Model file for the job. Use its own axes, mm. Face numbers are marked on the shaded views. A direction names the side the tool comes from. Give positions to 0.01 mm unless a question says otherwise; leave off trailing zeros. Loops run counter-clockwise (first coordinate to the right, second up) from the corner with the lowest first, then second, coordinate; pieces in that order, holes last. Notation, with made-up numbers: M 31,-39 L 88,-39 A26 cw 88,-11 Z; hole C 87.5,-12.75 d6. An arc over 180 degrees is marked long. Answer in a Markdown table with one row per item.
Autodesk Inventor part; units mm, degrees
ref_plane "YZ Plane" through (0, 0, 0) normal (1, 0, 0) x (0, 1, 0)
ref_plane "XZ Plane" through (0, 0, 0) normal (0, 1, 0) x (-1, 0, 0)
ref_plane "XY Plane" through (0, 0, 0) normal (0, 0, 1) x (1, 0, 0)
sketch "Sketch1" plane through (0, 0, 0) normal (0, 0, 1) x (1, 0, 0)
  line L0 (-119.142, 1.6299) -> (13.858, 1.6299)
  line L1 (14.858, 0.6299) -> (14.858, -42.3701)
  line L2 (13.858, -43.3701) -> (-119.142, -43.3701)
  line L3 (-120.142, -42.3701) -> (-120.142, 0.6299)
  arc A0 (-119.142, 1.6299) -> (-120.142, 0.6299) centre (-119.142, 0.6299) ccw
  arc A1 (-120.142, -42.3701) -> (-119.142, -43.3701) centre (-119.142, -42.3701) ccw
  arc A2 (13.858, -43.3701) -> (14.858, -42.3701) centre (13.858, -42.3701) ccw
  arc A3 (14.858, 0.6299) -> (13.858, 1.6299) centre (13.858, 0.6299) ccw
  circle A4 centre (8.858, -4.3701) radius 1.5
  circle A5 centre (-87.642, -37.3701) radius 1.5
  circle A6 centre (-75.642, -37.3701) radius 1.5
  circle A7 centre (8.858, -37.3701) radius 1.5
  circle A8 centre (-87.642, -4.3701) radius 1.5
  circle A9 centre (-75.642, -4.3701) radius 1.5
  point P0 (0, 0)
  point P1 (-120.142, 1.6299)
  point P2 (14.858, 1.6299)
  dimension "d0" = 135
  dimension "d2" = 1
  dimension "d3" = 1
  dimension "d7" = 3
  dimension "d8" = 6
  dimension "d9" = 6
  dimension "d10" = 3
  dimension "d11" = 3
  dimension "d14" = 3
  dimension "d15" = 6
  dimension "d16" = 6
  dimension "d17" = 6
  dimension "d18" = 6
  dimension "d19" = 12
  dimension "d20" = 32.5
  dimension "d21" = 3
  dimension "d22" = 3
  dimension "d23" = 6
  dimension "d24" = 6
  dimension "d25" = 32.5
  dimension "d26" = 12
extrude "Extrusion1" add sketch "Sketch1" along normal blind 1
sketch "Sketch2" plane through (14.858, -42.3701, 0) normal (1, 0, 0) x (0, 0, -1)
  line L0 (0, 44) -> (-1, 44)
  line L1 (-25, -1) -> (0, -1)
  line L2 (0, -1) -> (0, 44)
  line L3 (0, 44) -> (-25, 44)
  line L4 (-25, 44) -> (-25, -1)
  line L5 (0, 0) -> (0, -1)
  line L6 (0, -1) -> (-10, -1)
  line L7 (-10, -1) -> (-10, 44)
  line L8 (-10, 44) -> (0, 44)
  line L9 (0, 44) -> (0, -1)
  line L10 (0, -1) -> (-1, -1)
  line L11 (-1, -1) -> (-1, 44)
  line L12 (-1, 44) -> (0, 44)
  line L13 (0, 44) -> (0, -1)
  line L14 (-1, 0) -> (-1, 43)
  line L15 (-10, 9) -> (-1, 9)
  line L16 (-1, 9) -> (-1, 29)
  line L17 (-1, 29) -> (-10, 29)
  line L18 (-10, 29) -> (-10, 9)
  line L19 (-25, 5) -> (-10, 5)
  line L20 (-10, 5) -> (-10, 30)
  line L21 (-10, 30) -> (-25, 30)
  line L22 (-25, 30) -> (-25, 5)
  point P0 (0, 42.3701)
  point P1 (-1, 9)
  dimension "d29" = 25
  dimension "d30" = 10
  dimension "d31" = 10
  dimension "d32" = 20
  dimension "d33" = 6
  dimension "d34" = 25
extrude "Extrusion2" add sketch "Sketch2" against normal blind 1 contours L11 L17 L7 L3 | L7 L21 L4 L3 | L1 L7 L15 L11 | L1 L4 L19 L7
sketch "Sketch3" plane through (-119.142, -43.3701, 0) normal (0, -1, 0) x (1, 0, 0)
  line L0 (0, 0) -> (-1, 0)
  line L1 (134, 25) -> (134, 10)
  line L2 (-1, 0) -> (134, 0)
  line L3 (134, 0) -> (134, 25)
  line L4 (134, 25) -> (-1, 25)
  line L5 (-1, 25) -> (-1, 0)
  point P0 (119.142, 0)
extrude "Extrusion3" add sketch "Sketch3" against normal blind 1
sketch "Sketch4" plane through (-119.142, 1.6299, 0) normal (0, 1, 0) x (1, 0, 0)
  line L0 (134, -25) -> (134, -10)
  line L1 (-1, 0) -> (-1, -1)
  line L2 (134, -25) -> (-1, -25)
  line L3 (-1, -25) -> (-1, 0)
  line L4 (-1, 0) -> (134, 0)
  line L5 (134, 0) -> (134, -25)
  point P0 (119.142, 0)
sketch "Sketch5" plane through (-120.142, -43.3701, 0) normal (-1, 0, 0) x (0, 0, 1)
  line L0 (25, 45) -> (1, 45)
  line L1 (0, 44) -> (0, 0)
  line L2 (25, 45) -> (0, 45)
  line L3 (0, 45) -> (0, 0)
  line L4 (0, 0) -> (25, 0)
  line L5 (25, 0) -> (25, 45)
  circle A0 centre (8, 33) radius 2
  circle A1 centre (8, 8) radius 2
  point P0 (0, 43.3701)
  point P1 (1, 45)
  dimension "d39" = 25
  dimension "d40" = 12
  dimension "d42" = 8
  dimension "d47" = 4
  dimension "d48" = 4
  dimension "d49" = 8
extrude "Extrusion4" add sketch "Sketch5" against normal blind 2
extrude "Extrusion5" add sketch "Sketch4" against normal blind 1
properties part number "arduino mould"
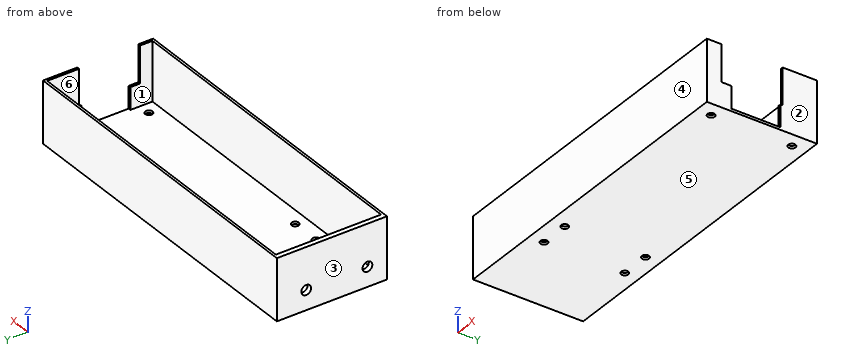
Q1. Probe probe 1 along Y at (x, z) = (-118.7, 8); probe 2 along X at (y, z) = (-5, 21); probe 3 along Y at (x, z) = (-72.5, 1.75). List the from-to ranges inside material, lowest first.
Reported:
| item | result |
|---|---|
| probe 1 | -43.37 to -37.37, -33.37 to -12.37, -8.37 to 1.63 |
| probe 2 | -120.14 to -118.14, 13.86 to 14.86 |
| probe 3 | -43.37 to -42.37, 0.63 to 1.63 |
Q2. Saw through at A-A (z = 8). Give the cut face in (x, y).
Reported:
| item | result |
|---|---|
| outline | M -120.14,-43.37 L 14.86,-43.37 L 14.86,-33.37 L 13.86,-33.37 L 13.86,-42.37 L -118.14,-42.37 L -118.14,-37.37 L -120.14,-37.37 Z; M -120.14,-33.37 L -118.14,-33.37 L -118.14,-12.37 L -120.14,-12.37 Z; M -120.14,-8.37 L -118.14,-8.37 L -118.14,0.63 L 13.86,0.63 L 13.86,-13.37 L 14.86,-13.37 L 14.86,1.63 L -120.14,1.63 Z |
Q3. 3-axis set-ups, long thin cutter, end or side, ignore diameter. For the marked faces 5 and 6: which of +Z, -Z, +X, -X, +Y, -Y reach the whole face in a straight line?
Reported:
| item | result |
|---|---|
| face 5 | -Z, +X, -X, +Y, -Y |
| face 6 | +Z |
Q4. Saw through at D-D (y = -26.5). Give the cut face in (x, z), and give its area (3 significant figures).
Reported:
| item | result |
|---|---|
| outline | M -120.14,0 L 14.86,0 L 14.86,1 L -118.14,1 L -118.14,25 L -120.14,25 Z |
| area | 183 mm² |
Q5. Saw through at B-B (z = 2.5). Give the cut face in (x, y), and give its area (3 significant figures).
Reported:
| item | result |
|---|---|
| outline | M -120.14,-43.37 L 14.86,-43.37 L 14.86,-33.37 L 13.86,-33.37 L 13.86,-42.37 L -118.14,-42.37 L -118.14,0.63 L 13.86,0.63 L 13.86,-13.37 L 14.86,-13.37 L 14.86,1.63 L -120.14,1.63 Z |
| area | 379 mm² |
Q6. Mould opens along X. For the marked faces 1, 2, 3 and 4 say: released by +X, released by -X, zero draft, split by the parting line, or undercut.
Reported:
| item | result |
|---|---|
| face 1 | undercut |
| face 2 | released by +X |
| face 3 | released by -X |
| face 4 | zero draft |
Q7. Drop flat-ended pins along their axis: pin 1 (8 mm diameter, centred on x = -59.5, y = -19, fed in from -Z); pin 2 (5 mm diameter, centred on x = 8.86, y = -4.37, fed in from +Z); pin 3 (2.5 mm diameter, centred on x = -87.64, y = -4.37, fed in from -Z). Give the stop position or say it passes through.
Reported:
| item | result |
|---|---|
| pin 1 | z = 0 |
| pin 2 | z = 1 |
| pin 3 | through |
Q8. Saw through at C-C (x = -104). Give the cut face in (y, z).
Reported:
| item | result |
|---|---|
| outline | M -43.37,0 L 1.63,0 L 1.63,25 L 0.63,25 L 0.63,1 L -42.37,1 L -42.37,25 L -43.37,25 Z |
